Build history of the part. All positions in model axes, mm. Face numbers are marked on the shaded views. A direction names the side the tool comes from. Coordinates: 2 decimals unless noted, no trailing zeros. Write each loop counter-clockwise with the first axis right and the second up, starting at its lowest first coordinate (ties: lowest second). Pieces come first, ordered by that corner, then holes.
```python
from build123d import *

# Parameters (mm, degrees)
F1_DEPTH = 25
F3_DEPTH = 2.5
F4_W     = 3.6095191927
F4_H     = 104.7
F5_DEPTH = 5.1
F6_DEPTH = 2.5


with BuildPart() as f1:
    # F0 (on Top) → F1 (new body)
    with BuildSketch(Plane.XY):
        Polygon((-21.9167374188, -55.3413778543), (-21.9167374188, -50.0413778543), (-25.5262566115, -50.0413778543), (-25.5262566115, -57.8413778543), (-12.9167374188, -57.8413778543), (-12.9167374188, -15.6176477188), (-12.9167374188, -9.371153079), (-12.9167374188, 34.286143216), (-12.9167374188, 54.6586221457), (-15.4167374188, 54.6586221457), (-15.4167374188, -55.3413778543), (-21.4532855898, -55.3413778543), align=None)
        Polygon((-12.9167374188, -9.371153079), (-12.9167374188, -15.6176477188), (25.1562967896, -57.8413778543), (30.7887457311, -57.8413778543), align=None)
    extrude(amount=F1_DEPTH)

    # F2 (on face) → F3 (join)
    with BuildSketch(Plane.XY.offset(25)):
        Polygon((-15.4167374188, -55.3413778543), (-15.4167374188, 54.6586221457), (-25.5262566115, 54.6586221457), (-25.5262566115, -50.0413778543), (-21.9167374188, -50.0413778543), (-21.9167374188, -55.3413778543), align=None)
        Polygon((-12.9167374188, -9.371153079), (-12.9167374188, 54.6586221457), (-15.4167374188, 54.6586221457), (-15.4167374188, -55.3413778543), (-21.9167374188, -55.3413778543), (-21.9167374188, -50.0413778543), (-25.5262566115, -50.0413778543), (-25.5262566115, -57.8413778543), (-12.9167374188, -57.8413778543), (-12.9167374188, -15.6176477188), align=None)
    extrude(amount=F3_DEPTH)

    # F4 (on face) → F5 (join)
    with BuildSketch(Plane(origin=(0, 0, 25), x_dir=(1, 0, 0), z_dir=(0, 0, -1))):
        with Locations((-23.7214970151, -2.3086221457)):
            Rectangle(F4_W, F4_H)
    extrude(amount=F5_DEPTH)

    # F6 (add, through all): a face of the model
    f6_faces = [f1.faces().sort_by_distance(p)[0] for p in [
        (7.5602195643, -35.1320371457, 25),
    ]]
    extrude(f6_faces, amount=F6_DEPTH)


solid = f1.part
```
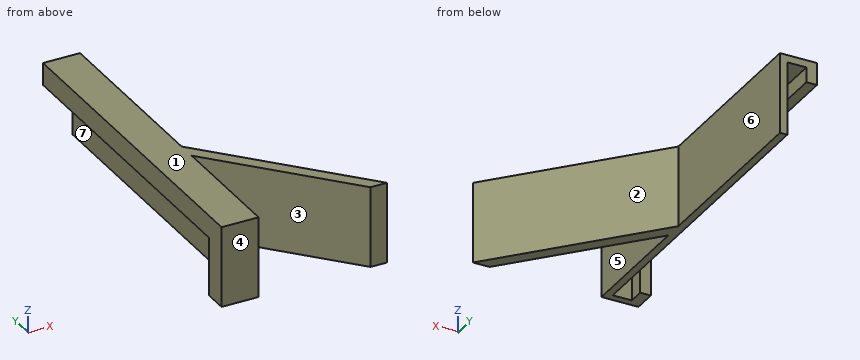
1. Probe line 1 along X through (y, z) = (-25, 21); line 2 along X through (y, z) = (-22.5, 22); line 3 along Z through (x, y) = (-18.5, -16.5). List the from-to ranges inside material, lowest first.
Computed values:
line 1: x = -25.53 to -21.92, -15.42 to -12.92, -4.46 to 1.18
line 2: x = -25.53 to -21.92, -15.42 to -12.92, -6.71 to -1.08
line 3: z = 25 to 27.5
2. Saw through at D-D on y = 5. List the corners of the cut face in (x, z).
Computed values:
outline: (-25.53, 19.9) - (-21.92, 19.9) - (-21.92, 25) - (-15.42, 25) - (-15.42, 0) - (-12.92, 0) - (-12.92, 27.5) - (-25.53, 27.5) - close
3. Saw through at A-A on y = -21.5. List the corners of the cut face in (x, z).
Computed values:
outline: (-25.53, 19.9) - (-21.92, 19.9) - (-21.92, 25) - (-15.42, 25) - (-15.42, 0) - (-12.92, 0) - (-12.92, 27.5) - (-25.53, 27.5) - close; (-7.61, 0) - (-1.98, 0) - (-1.98, 27.5) - (-7.61, 27.5) - close
4. Flat gauge pins, fed straight in: pin 1 (7.5 mm diameter, centred on y = -8.5, z = 8.5, fed in from -X); pin 2 (2 mm diameter, centred on x = -19, z = 17, fed in from +Y); pin 3 (3 mm diameter, centred on x = -23, y = -22.5, fed in from -Z). Where does each tip first touch, or does it go through?
Computed values:
pin 1: stops at x = -15.42
pin 2: stops at y = -55.34
pin 3: stops at z = 19.9
5. Saw through at B-B on z = 8.5. List the corners of the cut face in (x, y).
Computed values:
outline: (-25.53, -57.84) - (-12.92, -57.84) - (-12.92, -15.62) - (25.16, -57.84) - (30.79, -57.84) - (-12.92, -9.37) - (-12.92, 54.66) - (-15.42, 54.66) - (-15.42, -55.34) - (-21.92, -55.34) - (-21.92, -50.04) - (-25.53, -50.04) - close
6. 3-axis set-ups, long thin cutter, end or side, ignore diameter. For the marked faces 4, 5, 6 and 7: which of +Z, -Z, +X, -X, +Y, -Y reach the whole face in a straight line?
Computed values:
face 4: +Z, -Z, +X, -X, -Y
face 5: +Z, -Z, -Y
face 6: +Z, -Z, +X, +Y
face 7: -Z, +Y
7. Mould opens along X. For the marked faces 1, 2 and 3 say: +X half, -X half, draft (parallel to the pull), parting line (faces both ways), or undercut.
Computed values:
face 1: draft
face 2: +X half
face 3: undercut
8. Saw through at C-C on x = -20.5. List the corners of the cut face in (y, z).
Computed values:
outline: (-57.84, 0) - (-55.34, 0) - (-55.34, 25) - (54.66, 25) - (54.66, 27.5) - (-57.84, 27.5) - close
